Autodesk Inventor part; units mm, degrees
ref_plane "YZ Plane" through (0, 0, 0) normal (1, 0, 0) x (0, 1, 0)
ref_plane "XZ Plane" through (0, 0, 0) normal (0, 1, 0) x (-1, 0, 0)
ref_plane "XY Plane" through (0, 0, 0) normal (0, 0, 1) x (1, 0, 0)
sketch "Sketch1" plane through (0, 0, 0) normal (0, 1, 0) x (-1, 0, 0)
  line L0 (0, 0) -> (-170, 0)
  line L1 (-170, 0) -> (-170, -65)
  line L2 (-170, -65) -> (0, -65)
  line L3 (0, -65) -> (0, 0)
  line L4 (0, 0) -> (0, -20)
  line L5 (0, -20) -> (-20, -20)
  circle A0 centre (-20, -20) radius 4.5
  dimension "d0" = 170
  dimension "d1" = 65
  dimension "d2" = 20
  dimension "d3" = 20
  dimension "d4" = 9
extrude "Extrusion1" add sketch "Sketch1" along normal blind 15
properties part number "temp"
Can you work these out from the model? Positions are in its coordinate system, mm. Coordinates: 2 decimals unless noted, no trailing zeros. Order: outer loops, then holes, each group sorted by start corner. A loop starts at its lowest first (then second) coordinate and runs counter-clockwise, first axis right, second up. Notation, with made-up numbers: (-9, 69.25) - (4, 69.25) arc R24 cw to (4, 84.25) - close; hole circle Ø7 at (-34.5, -1.5). An arc over 180 degrees is marked (long way). Answer in a Markdown table with one row per item.
1. If I drill on line 1 along Z through (x, y) = (20, 9.5), over which ranges is the centre line in solid material (lowest first)?
Reply:
| item | result |
|---|---|
| line 1 | z = -65 to -24.5, -15.5 to 0 |
2. For pin 1 (8 mm diameter, centred on x = 20, z = -20, fed in from -Y), with a flat end and sliding along its axis, tell me the tip position at first contact or that it passes through.
Reply:
| item | result |
|---|---|
| pin 1 | passes through |
3. Suppose I cut it at B-B (x = 20). Please give me the cut outline in (y, z), and give its area (3 significant figures).
Reply:
| item | result |
|---|---|
| outline | (0, -65) - (15, -65) - (15, -24.5) - (0, -24.5) - close; (0, -15.5) - (15, -15.5) - (15, 0) - (0, 0) - close |
| area | 840 mm^2 |
4. If we mould it in two halves opening along Z, with no side actions, what happens to faces 1 (the flat face through (86, 7, -65)), 2 (the cylindrical face through (23.32, 7.4, -23.04)), 3 (the flat face through (0, 7, -33))? For each: pulls with the +Z half, pulls with the -Z half, needs draft (parallel to the pull), parting line crosses it, or undercut.
Reply:
| item | result |
|---|---|
| face 1 | pulls with the -Z half |
| face 2 | undercut |
| face 3 | needs draft |
5. Suppose I cut it at A-A (z = -20). Please give me the cut outline in (x, y), and give its area (4 significant figures).
Reply:
| item | result |
|---|---|
| outline | (0, 0) - (15.5, 0) - (15.5, 15) - (0, 15) - close; (24.5, 0) - (170, 0) - (170, 15) - (24.5, 15) - close |
| area | 2,415 mm^2 |
